```python
from build123d import *

# Parameters (mm, degrees)
SKETCH1_W           = 85
SKETCH1_H           = 120
BOSS_EXTRUDE1_DEPTH = 7
FILLET1_R           = 8
SKETCH2_W           = 64
SKETCH2_H           = 81
SKETCH2_W_2         = 61
SKETCH2_H_2         = 78
BOSS_EXTRUDE2_DEPTH = 6


with BuildPart() as part:
    # Sketch1 → Boss-Extrude1 (new body)
    with BuildSketch(Plane(origin=(0, 0, 0), x_dir=(1, 0, 0), z_dir=(0, 1, 0))):
        with Locations((42.5, 60)):
            Rectangle(SKETCH1_W, SKETCH1_H)
    extrude(amount=BOSS_EXTRUDE1_DEPTH)

    # Fillet1
    fillet1_edges = [part.edges().sort_by_distance(p)[0] for p in [
        (85, 3.5, 0),
        (0, 3.5, 0),
    ]]
    fillet(fillet1_edges, radius=FILLET1_R)

    # Sketch2 → Boss-Extrude2 (add)
    with BuildSketch(Plane(origin=(0, 7, 0), x_dir=(1, 0, 0), z_dir=(0, 1, 0))):
        with Locations((43, 64.739607224)):
            Rectangle(SKETCH2_W, SKETCH2_H)
        with Locations((43, 64.739607224)):
            Rectangle(SKETCH2_W_2, SKETCH2_H_2, mode=Mode.SUBTRACT)
    extrude(amount=BOSS_EXTRUDE2_DEPTH)


solid = part.part
```
CAD build for the part. Positions are in the model's coordinates, mm. A direction names the side the tool comes from. Round coordinates to 2 decimals unless told otherwise and drop trailing zeros. Write each loop counter-clockwise with the first axis right and the second up, starting at its lowest first coordinate (ties: lowest second). Pieces come first, ordered by that corner, then holes. Notation, with made-up numbers: (43.25, 48.5) - (88.25, 48.5) arc R26 ccw to (88.25, 77.5) - close; hole circle Ø6 at (89.25, -26). An arc over 180 degrees is marked (long way). Return JSON: item names as keys, results as strings. Group by question number.
Item 1: Mould opens along Z. For faces 1 (the face through (43, 10, -25.74)), 2 (the face through (82.594, 3.549, -2.281)), 3 (the face through (43, 13, -104)) say: +Z half, -Z half, draft (parallel to the pull), parting line (faces both ways), or undercut.
Item 2: Flat gauge pins, fed straight in: pin 1 Ø1.5 at (x, z) = (36.5, -33.5) entering from -Y; pin 2 Ø1.8 at (y, z) = (9.5, -59.5) entering from +X; pin 3 Ø3 at (y, z) = (9, -51) entering from -X; pin 4 Ø5 at (x, y) = (43.5, 10) entering from -Z. Where does each tip first touch, or does it go through?
Item 3: Band-saw the part on A-A on y = 8.75. List the corners of the cut face in (x, z), plus the area to 3 significant figures.
Item 4: 3-axis set-ups, long thin cutter, end or side, ignore diameter. For faces 4 (the face through (43, 10, -103.74)), 5 (the face through (11, 10, -64)), 6 (the face through (43, 10, -24.24)): which of +Z, -Z, +X, -X, +Y, -Y reach the whole face in a straight line?
Item 5: Probe probe 1 along X at (y, z) = (10, -34); probe 2 along Z at (x, y) = (53, 10.25); probe 3 along Y at (x, z) = (35, -18). List the from-to ranges inside material, lowest first.
Item 6: Band-saw the part on D-D on z = -107. List the corners of the cut face in (x, y).
Item 7: Band-saw the part on C-C on z = -36. List the corners of the cut face in (x, y).
Item 8: Band-saw the part on B-B on x = 68. List the corners of the cut face in (y, z), plus the area to 3 significant figures.
Resolved:
{
 "1": {"face 1": "undercut", "face 2": "+Z half", "face 3": "draft"},
 "2": {"pin 1": "stops at y = 0", "pin 2": "stops at x = 75", "pin 3": "stops at x = 11", "pin 4": "stops at z = -105.24"},
 "3": {"outline": "(11, -105.24) - (75, -105.24) - (75, -24.24) - (11, -24.24) - close; hole (12.5, -103.74) - (73.5, -103.74) - (73.5, -25.74) - (12.5, -25.74) - close", "area": "426 mm²"},
 "4": {"face 4": "+Y", "face 5": "+Z, -Z, -X, +Y", "face 6": "+Z, +X, -X, +Y"},
 "5": {"probe 1": "x = 11 to 12.5, 73.5 to 75", "probe 2": "z = -105.24 to -103.74, -25.74 to -24.24", "probe 3": "y = 0 to 7"},
 "6": {"outline": "(0, 0) - (85, 0) - (85, 7) - (0, 7) - close"},
 "7": {"outline": "(0, 0) - (85, 0) - (85, 7) - (75, 7) - (75, 13) - (73.5, 13) - (73.5, 7) - (12.5, 7) - (12.5, 13) - (11, 13) - (11, 7) - (0, 7) - close"},
 "8": {"outline": "(0, -120) - (7, -120) - (7, -105.24) - (13, -105.24) - (13, -103.74) - (7, -103.74) - (7, -25.74) - (13, -25.74) - (13, -24.24) - (7, -24.24) - (7, 0) - (0, 0) - close", "area": "858 mm²"}
}
